Can you work these out from the model? Positions are in its coordinate system, mm. Give positions to 0.01 mm unless a question says otherwise; leave off trailing zeros. Write each loop counter-clockwise with the first axis right and the second up, starting at its lowest first coordinate (ties: lowest second). Pieces come first, ordered by that corner, then holes. Notation, with made-up numbers: M 49.25,69.25 L 65.25,69.25 A9 cw 65.25,78.25 Z; hole C -13,-8 d6. An arc over 180 degrees is marked long. Write each question's results on one line, items separated by ' | '.
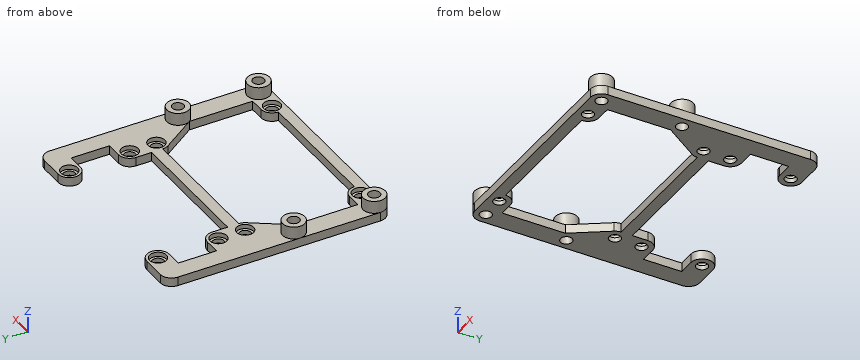
from build123d import *

# Parameters (mm, degrees)
F2_DEPTH = 2.54
F3_R     = 3.175
F4_DEPTH = 3.556
F5_R     = 1.651
F6_DEPTH = 6.096
F7_R     = 2.413
F8_DEPTH = 1.27


with BuildPart() as f2:
    # F1 (on Top) → F2 (new body)
    with BuildSketch(Plane.XY):
        with BuildLine():
            Line((-32.1691, 46.4058), (-32.1691, -11.5062))
            ThreePointArc((-32.1691, -11.5062), (-31.239164, -13.751264), (-28.9941, -14.6812))
            Line((-28.9941, -14.6812), (28.9941, -14.6812))
            ThreePointArc((28.9941, -14.6812), (31.239164, -13.751264), (32.1691, -11.5062))
            Line((32.1691, -11.5062), (32.1691, 46.4058))
            ThreePointArc((32.1691, 46.4058), (31.239164, 48.650864), (28.9941, 49.5808))
            Line((28.9941, 49.5808), (22.225, 49.5808))
            ThreePointArc((22.225, 49.5808), (19.05, 46.4058), (22.225, 43.2308))
            Line((22.225, 43.2308), (26.797, 43.2308))
            Line((26.797, 43.2308), (26.797, 32.3088))
            Line((26.797, 32.3088), (22.225, 32.3088))
            ThreePointArc((22.225, 32.3088), (19.979936, 31.378864), (19.05, 29.1338))
            Line((19.05, 29.1338), (19.05, 24.6888))
            Line((19.05, 24.6888), (-19.05, 24.6888))
            Line((-19.05, 24.6888), (-19.05, 29.1338))
            ThreePointArc((-19.05, 29.1338), (-19.979936, 31.378864), (-22.225, 32.3088))
            Line((-22.225, 32.3088), (-26.797, 32.3088))
            Line((-26.797, 32.3088), (-26.797, 43.2308))
            Line((-26.797, 43.2308), (-22.225, 43.2308))
            ThreePointArc((-22.225, 43.2308), (-19.05, 46.4058), (-22.225, 49.5808))
            Line((-22.225, 49.5808), (-28.9941, 49.5808))
            ThreePointArc((-28.9941, 49.5808), (-31.239164, 48.650864), (-32.1691, 46.4058))
        make_face()
        with BuildLine():
            Line((-26.364209, 9.727352), (-19.595109, 19.734952))
            ThreePointArc((-19.595109, 19.734952), (-19.189335, 20.583552), (-19.05, 21.5138))
            Line((-19.05, 21.5138), (19.05, 21.5138))
            ThreePointArc((19.05, 21.5138), (19.189335, 20.583552), (19.595109, 19.734952))
            Line((19.595109, 19.734952), (26.364209, 9.727352))
            Line((26.364209, 9.727352), (26.364209, -8.3312))
            Line((26.364209, -8.3312), (22.225, -8.3312))
            ThreePointArc((22.225, -8.3312), (19.979936, -9.261136), (19.05, -11.5062))
            Line((19.05, -11.5062), (-19.05, -11.5062))
            ThreePointArc((-19.05, -11.5062), (-19.979936, -9.261136), (-22.225, -8.3312))
            Line((-22.225, -8.3312), (-26.364209, -8.3312))
            Line((-26.364209, -8.3312), (-26.364209, 9.727352))
        make_face(mode=Mode.SUBTRACT)
    extrude(amount=F2_DEPTH)

    # F3 (on face) → F4 (join)
    with BuildSketch(Plane.XY.offset(2.54)):
        with Locations((-28.9941, -11.5062)):
            Circle(F3_R)
        with Locations((-28.9941, 11.5062)):
            Circle(F3_R)
        with Locations((28.9941, 11.5062)):
            Circle(F3_R)
        with Locations((28.9941, -11.5062)):
            Circle(F3_R)
    extrude(amount=F4_DEPTH)

    # F5 (on face) → F6 (cut, through all)
    with BuildSketch(Plane(origin=(0, 0, 0), x_dir=(1, 0, 0), z_dir=(0, 0, -1))):
        with Locations((28.9941, -11.5062)):
            Circle(F5_R)
        with Locations((22.225, -21.5138)):
            Circle(F5_R)
        with Locations((-22.225, -21.5138)):
            Circle(F5_R)
        with Locations((-28.9941, -11.5062)):
            Circle(F5_R)
        with Locations((-28.9941, 11.5062)):
            Circle(F5_R)
        with Locations((-22.225, 11.5062)):
            Circle(F5_R)
        with Locations((22.225, 11.5062)):
            Circle(F5_R)
        with Locations((28.9941, 11.5062)):
            Circle(F5_R)
        with Locations((22.225, -29.1338)):
            Circle(F5_R)
        with Locations((22.225, -46.4058)):
            Circle(F5_R)
        with Locations((-22.225, -29.1338)):
            Circle(F5_R)
        with Locations((-22.225, -46.4058)):
            Circle(F5_R)
    extrude(amount=-F6_DEPTH, mode=Mode.SUBTRACT)

    # F7 (on face) → F8 (cut)
    with BuildSketch(Plane.XY.offset(2.54)):
        with Locations((22.225, -11.5062)):
            Circle(F7_R)
        with Locations((22.225, 21.5138)):
            Circle(F7_R)
        with Locations((22.225, 29.1338)):
            Circle(F7_R)
        with Locations((22.225, 46.4058)):
            Circle(F7_R)
        with Locations((-22.225, 46.4058)):
            Circle(F7_R)
        with Locations((-22.225, 29.1338)):
            Circle(F7_R)
        with Locations((-22.225, 21.5138)):
            Circle(F7_R)
        with Locations((-22.225, -11.5062)):
            Circle(F7_R)
    extrude(amount=-F8_DEPTH, mode=Mode.SUBTRACT)


solid = f2.part
Item 1: If I drill on line 1 (Y direction, x = -18, z = 1); line 2 (X direction, y = 0, z = 0.75); line 3 (X direction, y = 40, z = 2.25), over which ranges is the centre line in solid material (lowest first)? Write a range as from..to.
Geometry says:
line 1: y = -14.68..-11.51, 21.51..24.69 | line 2: x = -32.17..-26.36, 26.36..32.17 | line 3: x = -32.17..-26.8, 26.8..32.17
Item 2: I'm going to push flat-ended pins straight in: pin 1 (4 mm diameter, centred on x = -22.22, y = 29.13, fed in from +Z); pin 2 (3 mm diameter, centred on x = 22.22, y = 46.41, fed in from -Z); pin 3 (12 mm diameter, centred on x = 3, y = 30, fed in from +Z). Where does each tip first touch, or does it pass through?
Geometry says:
pin 1: stops at z = 1.27 | pin 2: passes through | pin 3: stops at z = 2.54
Item 3: I want a section at D-D, the plane y = 30. Please give me the cut outline in (x, z), and give its area (3 significant figures).
Geometry says:
outline: M -32.17,0 L -23.63,0 L -23.63,1.27 L -24.48,1.27 L -24.48,2.54 L -32.17,2.54 Z; M -20.82,0 L -19.17,0 L -19.17,2.54 L -19.97,2.54 L -19.97,1.27 L -20.82,1.27 Z; M 19.17,0 L 20.82,0 L 20.82,1.27 L 19.97,1.27 L 19.97,2.54 L 19.17,2.54 Z; M 23.63,0 L 32.17,0 L 32.17,2.54 L 24.48,2.54 L 24.48,1.27 L 23.63,1.27 Z | area: 47.5 mm2
Item 4: I want a section at B-B, the plane z = 4.75. Please give me the cut outline in (x, y) (3 decimals).
Geometry says:
outline: C -28.994,-11.506 d6.35; C -28.994,11.506 d6.35; C 28.994,-11.506 d6.35; C 28.994,11.506 d6.35; hole C -28.994,-11.506 d3.302; hole C -28.994,11.506 d3.302; hole C 28.994,-11.506 d3.302; hole C 28.994,11.506 d3.302
Item 5: I want a section at C-C, the plane x = -1.5. Please give me the cut outline in (y, z), and give its area (3 significant figures).
Geometry says:
outline: M -14.68,0 L -11.51,0 L -11.51,2.54 L -14.68,2.54 Z; M 21.51,0 L 24.69,0 L 24.69,2.54 L 21.51,2.54 Z | area: 16.1 mm2
Item 6: I want a section at A-A, the plane y = 41. Please give me the cut outline in (x, z), and give its area (3 significant figures).
Geometry says:
outline: M -32.17,0 L -26.8,0 L -26.8,2.54 L -32.17,2.54 Z; M 26.8,0 L 32.17,0 L 32.17,2.54 L 26.8,2.54 Z | area: 27.3 mm2
